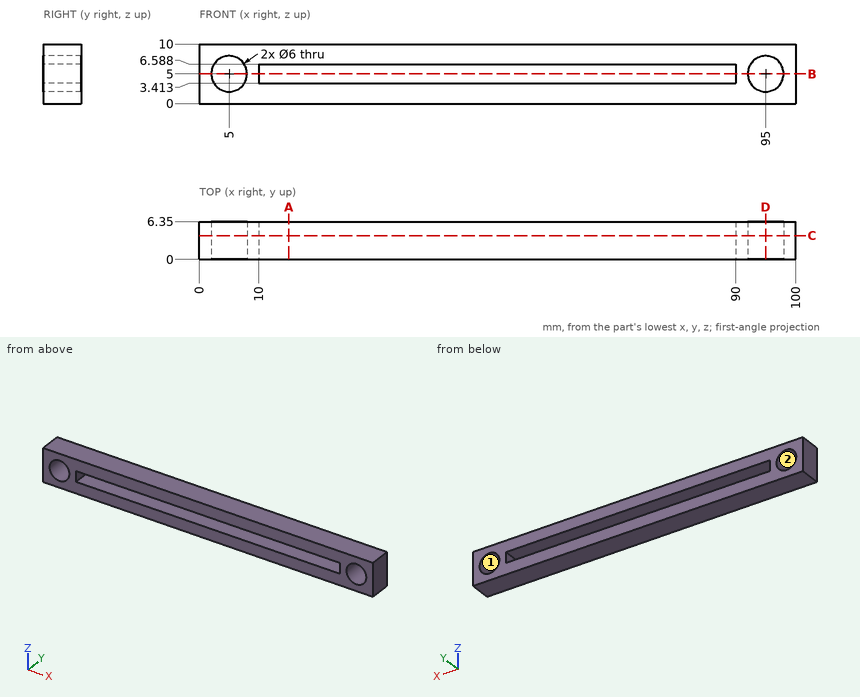
Can you work these out from the drawing? Everything is in mm from the part's minimum corner. Give positions to 0.01 mm unless a question says otherwise; leave off trailing zeros. Loops run counter-clockwise (first coordinate to the right, second up) from the corner with the lowest first, then second, coordinate; pieces in that order, holes last. Notation, with made-up numbers: (10.5, -20.5) -> (45.5, -20.5) arc R10 ccw to (45.5, -5.5) -> close; hole circle Ø5 at (48.25, -37). An arc over 180 degrees is marked (long way). Write item = value, one per line.
1) Thinking about a two-plate mould opening in Z: for the marked faces 1 and 2, which applies, released by +Z, released by -Z, zero draft, split by the parting line, or undercut?
Check result:
face_1 = undercut
face_2 = undercut
2) Suppose I cut it at D-D on x = 95. Write out the boundary of the cut face in (y, z).
Check result:
outline = (0, 0) -> (6.35, 0) -> (6.35, 2) -> (0, 2) -> close; (0, 8) -> (6.35, 8) -> (6.35, 10) -> (0, 10) -> close
3) Suppose I cut it at A-A on x = 15. Write out the boundary of the cut face in (y, z).
Check result:
outline = (0, 0) -> (6.35, 0) -> (6.35, 3.41) -> (0, 3.41) -> close; (0, 6.59) -> (6.35, 6.59) -> (6.35, 10) -> (0, 10) -> close
4) Suppose I cut it at C-C on y = 4. Write out the boundary of the cut face in (x, z).
Check result:
outline = (0, 0) -> (100, 0) -> (100, 10) -> (0, 10) -> close; hole circle Ø6 at (5, 5); hole (10, 3.41) -> (90, 3.41) -> (90, 6.59) -> (10, 6.59) -> close; hole circle Ø6 at (95, 5)
5) Will this pin go through, and if not, where does the flat tip stop? pin 1 (6 mm diameter, centred on x = 81, z = 5.5, fed in from +Y).
Check result:
pin_1 = 6.35
6) Suppose I cut it at B-B on z = 5. Write out the boundary of the cut face in (x, y).
Check result:
outline = (0, 0) -> (2, 0) -> (2, 6.35) -> (0, 6.35) -> close; (8, 0) -> (10, 0) -> (10, 6.35) -> (8, 6.35) -> close; (90, 0) -> (92, 0) -> (92, 6.35) -> (90, 6.35) -> close; (98, 0) -> (100, 0) -> (100, 6.35) -> (98, 6.35) -> close
7) I need wall thicknesses on L1, parallel to Z at x = 61.5, y = 0.5; L2, parallel to Z at x = 5, y = 1.75; L3, parallel to X at y = 4.5, z = 6.25. Which ranges of each line are inside material? Lowest first, please. Write a range as from..to.
Check result:
L1 = 0..3.41, 6.59..10
L2 = 0..2, 8..10
L3 = 0..2.27, 7.73..10, 90..92.27, 97.73..100
